```python
from build123d import *

# Parameters (mm, degrees)
SKETCH032_R   = 64.432756
PAD008_DEPTH  = 2
SKETCH033_R   = 44.95
SKETCH033_R_2 = 43.75
PAD009_DEPTH  = 36.4
FILLET009_R   = 0.99
FILLET010_R   = 2.5


with BuildPart() as part:
    # Sketch032 → Pad008 (new body)
    with BuildSketch(Plane.XY):
        Circle(SKETCH032_R)
    extrude(amount=PAD008_DEPTH)

    # Sketch033 → Pad009 (join)
    with BuildSketch(Plane.XY.offset(2)):
        Circle(SKETCH033_R)
        Circle(SKETCH033_R_2, mode=Mode.SUBTRACT)
    extrude(amount=PAD009_DEPTH)

    # Fillet009
    fillet009_edges = [part.edges().sort_by_distance(p)[0] for p in [
        (-44.95, 0, 38.4),
        (-64.432756, 0, 2),
        (-64.432756, 0, 0),
    ]]
    fillet(fillet009_edges, radius=FILLET009_R)

    # Fillet010
    fillet010_edges = [part.edges().sort_by_distance(p)[0] for p in [
        (-43.75, 0, 2),
    ]]
    fillet(fillet010_edges, radius=FILLET010_R)


solid = part.part
```
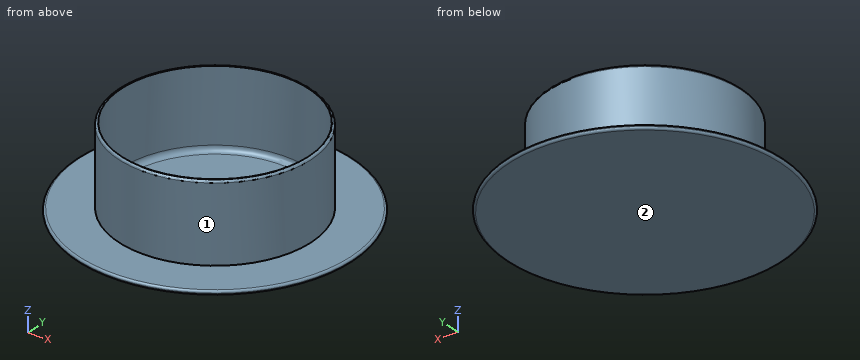
Verification items for the finished model (mm, model axes). Face numbers are marked on the shaded views. A direction names the side the tool comes from. Coordinates: 2 decimals unless noted, no trailing zeros. Loops run counter-clockwise (first coordinate to the right, second up) from the corner with the lowest first, then second, coordinate; pieces in that order, holes last. Notation, with made-up numbers: (58, -15) -> (79, -15) arc R9 cw to (79, -7) -> close; hole circle Ø3 at (21.5, 49.5). An arc over 180 degrees is marked (long way). Put each result on its own line as item: value.
1. Section check B-B, the plane z = 9. Record the boundary of the cut face in (x, y).
Result set:
outline: circle Ø89.9 at (0, 0); hole circle Ø87.5 at (0, 0)
2. Gauge pin test, flat ends, axial feed: P1, Ø3, axis at x = 20.5, y = 32.5, coming from the +Z side; P2, Ø5, axis at x = 13.5, z = 30, coming from the -Y side; P3, Ø8, axis at x = -2, z = 7, coming from the -Y side. Record the tip position at first contact, or that the pin passes through.
Result set:
P1: stops at z = 2
P2: stops at y = -43.58
P3: stops at y = -44.95
3. Thickness scan on line 1 (Y direction, x = 0, z = 12); line 2 (Z direction, x = -7.5, y = -40); line 3 (X direction, y = 20, z = 36.5). Record the ranges inside material, lowest first.
Result set:
line 1: y = -44.95 to -43.75, 43.75 to 44.95
line 2: z = 0 to 2
line 3: x = -40.26 to -38.91, 38.91 to 40.26
4. Tool access check on the marked faces 1 and 2. Record the directions out of +Z, -Z, +X, -X, +Y, -Y that give a thin tool (end or side, any length) a straight path to the whole face; none if there is none.
Result set:
face 1: +Z
face 2: -Z, +X, -X, +Y, -Y
